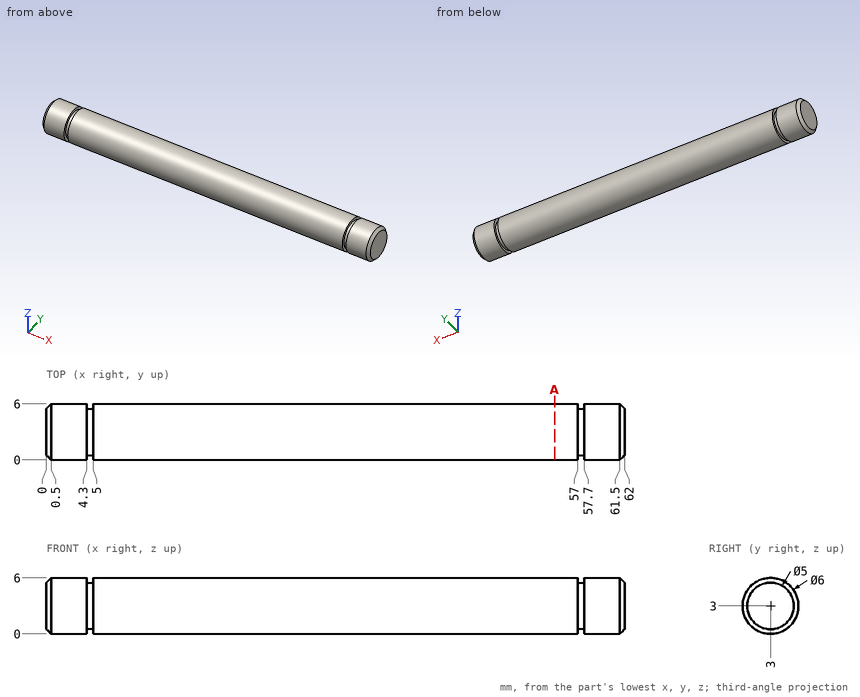
Answer from the drawing. Dimensions are ordinates in mm from the lowest x, y and z of the part. Coordinates: 2 decimals unless noted, no trailing zeros. Loops run counter-clockwise (first coordinate to the right, second up) from the corner with the lowest first, then second, coordinate; pieces in that order, holes last.
Q1. The part is cut by section A-A on x = 54.5. Write down the section's boundary in (y, z).
Q2. This flat-tipped pin is pushed along its axis until it touches: pin 1 Ø1 at (x, z) = (30, 0.5) entering from -Y. Where does it stop, or does it pass through?
Q3. Consider probe 1 along X at (y, z) = (3.85, 0.6); probe 2 along X at (y, z) = (5.4, 4.7); probe 3 along Y at (x, z) = (52, 3.25). Determine where each line is inside the solid, lowest interval first.
Results below:
1. outline: circle Ø6 at (3, 3)
2. pin 1: stops at y = 0.76
3. probe 1: x = 0.05 to 4.3, 5 to 57, 57.7 to 61.95
3. probe 2: x = 0.44 to 4.3, 5 to 57, 57.7 to 61.56
3. probe 3: y = 0.01 to 5.99
